```python
from build123d import *

# Parameters (mm, degrees)
F2_DEPTH = 467.36
F0_W     = 1740.8808469772
F0_H     = 2259.9012851715
F3_DEPTH = 60.96
F4_SCALE = 4.0036646816


with BuildPart() as f2:
    # F1 (on Top) → F2 (new body, symmetric)
    with BuildSketch(Plane.XY):
        with BuildLine():
            ThreePointArc((43.9515819812, 10.727503337), (23.9174424667, 1.374675553), (2.0415819812, -1.8329499959))
            Line((2.0415819812, -1.8329499959), (2.0415819812, -2.6877246239))
            ThreePointArc((2.0415819812, -2.6877246239), (24.6495492784, 0.7433272272), (45.2215819812, 10.727503337))
            Line((45.2215819812, 10.727503337), (43.9515819812, 10.727503337))
        make_face()
        with BuildLine():
            Line((2.0415819812, -2.6877246239), (2.0415819812, -1.8329499959))
            ThreePointArc((2.0415819812, -1.8329499959), (-19.8342785043, 1.374675553), (-39.8684180188, 10.727503337))
            Line((-39.8684180188, 10.727503337), (-41.1384180188, 10.727503337))
            ThreePointArc((-41.1384180188, 10.727503337), (-20.566385316, 0.7433272272), (2.0415819812, -2.6877246239))
        make_face()
    extrude(amount=F2_DEPTH, both=True)

    # F0 (on Front) → F3 (cut, symmetric)
    with BuildSketch(Plane.XZ):
        with Locations((133.3307623863, -204.713344574)):
            Rectangle(F0_W, F0_H)
        with BuildLine():
            Line((-1.295193345, -63.3309016509), (-1.295193345, 3.4090982191))
            Line((-1.295193345, 3.4090982191), (-0.065193265, 3.4090982191))
            Line((-0.065193265, 3.4090982191), (-0.065193265, -85.1709024209))
            Line((-0.065193265, -85.1709024209), (3.0674625036, -90.2881598735))
            Line((3.0674625036, -90.2881598735), (0.2766351171, -105.037851818))
            add(Edge.make_bspline(
                [(-0.680193305, -107.4909024849), (-0.3650057018, -107.493656038), (-0.0441852923, -106.265753928), (0.2766351171, -105.037851818)],
                knots=[0.5054719927, 0.5054719927, 0.5054719927, 0.5054719927, 1, 1, 1, 1], degree=3))
            add(Edge.make_bspline(
                [(-1.6349118244, -104.9110038356), (-1.3186339428, -106.1995459155), (-1.0023560613, -107.4880879954), (-0.680193305, -107.4909024849)],
                knots=[0, 0, 0, 0, 0.5054719927, 0.5054719927, 0.5054719927, 0.5054719927], degree=3))
            Line((-1.6349118244, -104.9110038356), (-4.5669513225, -90.2003612126))
            Line((-4.5669513225, -90.2003612126), (-1.295193345, -85.1709024209))
            Line((-1.295193345, -85.1709024209), (-1.295193345, -70.5809023909))
            Line((-1.295193345, -70.5809023909), (-4.495186945, -70.5809023909))
            Line((-4.495186945, -70.5809023909), (-4.495186945, -63.3309016509))
            Line((-4.495186945, -63.3309016509), (-1.295193345, -63.3309016509))
        make_face(mode=Mode.SUBTRACT)
        with BuildLine():
            Line((-0.680193305, -107.4909024849), (-0.680193305, -104.9110038356))
            Line((-0.680193305, -104.9110038356), (-1.6349118244, -104.9110038356))
            add(Edge.make_bspline(
                [(-1.6349118244, -104.9110038356), (-1.3186339428, -106.1995459155), (-1.0023560613, -107.4880879954), (-0.680193305, -107.4909024849)],
                knots=[0, 0, 0, 0, 0.5054719927, 0.5054719927, 0.5054719927, 0.5054719927], degree=3))
        make_face()
        with BuildLine():
            Line((0.2766351171, -105.037851818), (-0.680193305, -104.9110038356))
            Line((-0.680193305, -104.9110038356), (-0.680193305, -107.4909024849))
            add(Edge.make_bspline(
                [(-0.680193305, -107.4909024849), (-0.3650057018, -107.493656038), (-0.0441852923, -106.265753928), (0.2766351171, -105.037851818)],
                knots=[0.5054719927, 0.5054719927, 0.5054719927, 0.5054719927, 1, 1, 1, 1], degree=3))
        make_face()
    extrude(amount=F3_DEPTH, both=True, mode=Mode.SUBTRACT)


with BuildPart() as f2_1:
    # F4: moved
    add(f2.part.scale(F4_SCALE))


solid = f2_1.part
```
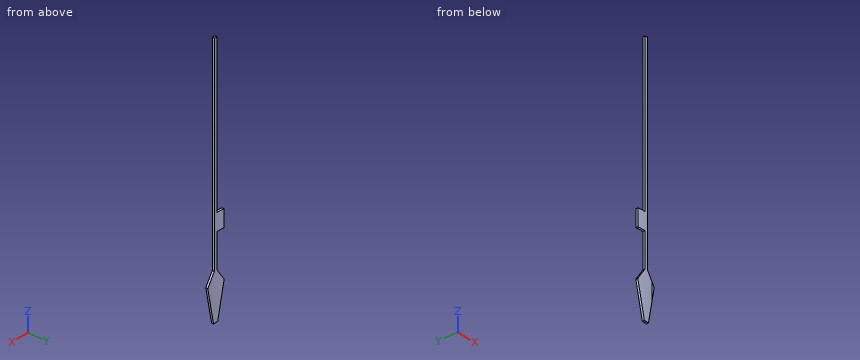
Build history of the part. All positions in model axes, mm. Give positions to 0.01 mm unless a question says otherwise; leave off trailing zeros. Loops run counter-clockwise (first coordinate to the right, second up) from the corner with the lowest first, then second, coordinate; pieces in that order, holes last.
1) Band-saw the part on A-A on y = -8.5. List the corners of the cut face in (x, z), then the cut area to 3 significant figures.
Values follow:
outline: (-18.28, -361.13) - (-6.55, -420.03) - (-2.72, -420.03) - (1.11, -420.54) - (12.28, -361.48) - (-0.26, -341) - (-0.26, 13.65) - (-5.19, 13.65) - (-5.19, -253.56) - (-18, -253.56) - (-18, -282.58) - (-5.19, -282.58) - (-5.19, -341) - close
area: 3,600 mm2
2) Drop flat-ended pins along their axis: P1, Ø2, axis at x = -14.5, y = -7.5, coming from the +Z side; P2, Ø1, axis at y = -8, z = -268, coming from the -X side; P3, Ø1.8, axis at x = -4.5, y = -9.5, coming from the -Z side. Give the stop position or say it passes through.
Values follow:
P1: stops at z = -253.56
P2: stops at x = -18
P3: stops at z = -420.03
3) Band-saw the part on C-C on z = -104. List the corners of the cut face in (x, y), then the cut area to 3 significant figures.
Values follow:
outline: (-5.19, -10.47) arc R305.08 ccw to (-0.26, -10.64) - (-0.26, -7.22) arc R305.08 cw to (-5.19, -7.05) - close
area: 16.9 mm2
4) Band-saw the part on D-D on z = -273. List the corners of the cut face in (x, y).
Values follow:
outline: (-18, -9.64) arc R305.08 ccw to (-0.26, -10.64) - (-0.26, -7.22) arc R305.08 cw to (-18, -6.21) - close
5) Probe line 1 along Y through (x, z) = (1, -371); line 2 along X through (y, z) = (-9.35, -120); line 3 along Y through (x, z) = (-2, -29.5). List the from-to ranges inside material, lowest first.
Values follow:
line 1: y = -10.68 to -7.25
line 2: x = -5.19 to -0.26
line 3: y = -10.59 to -7.17
6) Band-saw the part on B-B on x = -14.5. List the corners of the cut face in (y, z), then the cut area to 3 significant figures.
Values follow:
outline: (-9.92, -380.12) - (-6.49, -380.12) - (-6.49, -355.31) - (-9.92, -355.31) - close; (-9.92, -282.58) - (-6.49, -282.58) - (-6.49, -253.56) - (-9.92, -253.56) - close
area: 184 mm2
